Source: CAD feature listing. Evaluate the final solid. Frame: model axes, mm. A direction names the side the tool comes from. Give positions to 0.01 mm unless a question says otherwise; leave off trailing zeros. Order: outer loops, then holes, each group sorted by start corner. A loop starts at its lowest first (then second) coordinate and runs counter-clockwise, first axis right, second up. Notation, with made-up numbers: (47.5, -28.75) - (93.5, -28.75) arc R10 ccw to (93.5, -17.75) - close; hole circle Ø6 at (-24.75, 19.25). An arc over 180 degrees is marked (long way). Write each question's results on one line, items separated by ' | '. Start each with the question number.
Item 1: Mould query, pull axis Y, two halves, no side actions, for faces 1 (the flat face through (6, 29, 148)), 2 (the flat face through (0, 30, 148)), 3 (the flat face through (0, 18.7, 148)), 4 (the flat face through (-13.1, 15, 148)). Classes: released by +Y, released by -Y, zero draft, split by the parting line, or undercut.
Item 2: Contact query for flat-ended pins moving along their axis: pin 1 Ø9 at (x, z) = (-3.5, 187) entering from -Y; pin 2 Ø6 at (x, y) = (8.5, 13) entering from -Z; pin 3 Ø1.5 at (x, z) = (-6.5, 176) entering from +Y. Output: stop coordinate, or through.
Item 3: Section A-A on x = 6.25. Output: boundary loops of the cut face in (y, z).
Item 4: Section B-B on y = 8.5. Output: boundary loops of the cut face in (x, z), and give its area (3 significant figures).
Item 5: Set-up query: faces 5 (the flat face through (12.7, 15.3, 300)), 6 (the flat face through (-6, 29, 148)). Return all of +Z, -Z, +X, -X, +Y, -Y with unobstructed straight access to the full face (end or side cutting, diameter ignored); none if empty.
Item 6: Line query: line 1 along Y through (x, z) = (11.25, 179.5); line 2 along X through (y, z) = (2, 135); line 3 along Y through (x, z) = (-8.5, 126). Output: solid intervals per line, ascending.
```python
from build123d import *

# Parameters (mm, degrees)
BOSS_EXTRUDE1_DEPTH = 300


with BuildPart() as part:
    # Sketch1 → Boss-Extrude1 (new body)
    with BuildSketch(Plane.XY):
        with BuildLine():
            Line((-12.008392022, 30), (12.008392022, 30))
            ThreePointArc((12.008392022, 30), (12.072941744, 30.023623738), (12.106993351, 30.083333333))
            ThreePointArc((12.106993351, 30.083333333), (12.64181313, 30.498248595), (13.1, 30))
            Line((13.1, 30), (13.1, 17.7))
            Line((13.1, 17.7), (13.1, 0.4))
            ThreePointArc((13.1, 0.4), (12.982842712, 0.117157288), (12.7, 0))
            Line((12.7, 0), (10.9, 0))
            Line((10.9, 0), (10.9, 2))
            ThreePointArc((10.9, 2), (11.148496927, 2.248496927), (11.396993855, 2))
            Line((11.396993855, 2), (11.396993855, 1.4))
            ThreePointArc((11.396993855, 1.4), (11.514151142, 1.117157288), (11.796993855, 1))
            Line((11.796993855, 1), (11.996993855, 1))
            ThreePointArc((11.996993855, 1), (12.279836567, 1.117157288), (12.396993855, 1.4))
            Line((12.396993855, 1.4), (12.396993855, 2.441856285))
            ThreePointArc((12.396993855, 2.441856285), (12.3928338, 2.499395297), (12.380440165, 2.555737483))
            Line((12.380440165, 2.555737483), (12.11655369, 3.444262517))
            ThreePointArc((12.11655369, 3.444262517), (12.104160055, 3.500604703), (12.1, 3.558143715))
            Line((12.1, 3.558143715), (12.1, 17.3))
            ThreePointArc((12.1, 17.3), (11.982842712, 17.582842712), (11.7, 17.7))
            Line((11.7, 17.7), (-11.7, 17.7))
            ThreePointArc((-11.7, 17.7), (-11.982842712, 17.582842712), (-12.1, 17.3))
            Line((-12.1, 17.3), (-12.1, 3.558143715))
            ThreePointArc((-12.1, 3.558143715), (-12.104160055, 3.500604703), (-12.11655369, 3.444262517))
            Line((-12.11655369, 3.444262517), (-12.380440165, 2.555737483))
            ThreePointArc((-12.380440165, 2.555737483), (-12.3928338, 2.499395297), (-12.396993855, 2.441856285))
            Line((-12.396993855, 2.441856285), (-12.396993855, 1.4))
            ThreePointArc((-12.396993855, 1.4), (-12.279836567, 1.117157288), (-11.996993855, 1))
            Line((-11.996993855, 1), (-11.796993855, 1))
            ThreePointArc((-11.796993855, 1), (-11.514151142, 1.117157288), (-11.396993855, 1.4))
            Line((-11.396993855, 1.4), (-11.396993855, 2))
            ThreePointArc((-11.396993855, 2), (-11.148496927, 2.248496927), (-10.9, 2))
            Line((-10.9, 2), (-10.9, 0))
            Line((-10.9, 0), (-12.7, 0))
            ThreePointArc((-12.7, 0), (-12.982842712, 0.117157288), (-13.1, 0.4))
            Line((-13.1, 0.4), (-13.1, 17.7))
            Line((-13.1, 17.7), (-13.1, 30))
            ThreePointArc((-13.1, 30), (-12.64181313, 30.498248595), (-12.106993351, 30.083333333))
            ThreePointArc((-12.106993351, 30.083333333), (-12.072941744, 30.023623738), (-12.008392022, 30))
        make_face()
        with BuildLine():
            Line((-12.1, 28.6), (-12.1, 24.889865053))
            ThreePointArc((-12.1, 24.889865053), (-11.6, 24.02383965), (-12.1, 23.157814246))
            Line((-12.1, 23.157814246), (-12.1, 19.1))
            ThreePointArc((-12.1, 19.1), (-11.982842712, 18.817157288), (-11.7, 18.7))
            Line((-11.7, 18.7), (11.7, 18.7))
            ThreePointArc((11.7, 18.7), (11.982842712, 18.817157288), (12.1, 19.1))
            Line((12.1, 19.1), (12.1, 23.157814246))
            ThreePointArc((12.1, 23.157814246), (11.6, 24.02383965), (12.1, 24.889865053))
            Line((12.1, 24.889865053), (12.1, 28.6))
            ThreePointArc((12.1, 28.6), (11.982842712, 28.882842712), (11.7, 29))
            Line((11.7, 29), (0.173205081, 29))
            Line((0.173205081, 29), (0, 29.3))
            Line((0, 29.3), (-0.173205081, 29))
            Line((-0.173205081, 29), (-11.7, 29))
            ThreePointArc((-11.7, 29), (-11.982842712, 28.882842712), (-12.1, 28.6))
        make_face(mode=Mode.SUBTRACT)
    extrude(amount=BOSS_EXTRUDE1_DEPTH)


solid = part.part
```
Evaluation:
1) face 1: undercut | face 2: released by +Y | face 3: undercut | face 4: zero draft
2) pin 1: stops at y = 17.7 | pin 2: passes through | pin 3: stops at y = 30
3) outline: (17.7, 0) - (18.7, 0) - (18.7, 300) - (17.7, 300) - close; (29, 0) - (30, 0) - (30, 300) - (29, 300) - close
4) outline: (-13.1, 0) - (-12.1, 0) - (-12.1, 300) - (-13.1, 300) - close; (12.1, 0) - (13.1, 0) - (13.1, 300) - (12.1, 300) - close | area: 600 mm^2
5) face 5: +Z, +X, -X, +Y, -Y | face 6: +Z, -Z
6) line 1: y = 0 to 2.23, 17.7 to 18.7, 29 to 30 | line 2: x = -13.1 to -12.4, -11.4 to -10.9, 10.9 to 11.4, 12.4 to 13.1 | line 3: y = 17.7 to 18.7, 29 to 30
